Read the model definition and answer for the solid it produces. Units are mm, in the model's axes. A direction names the side the tool comes from. Round coordinates to 2 decimals unless told otherwise and drop trailing zeros. Order: outer loops, then holes, each group sorted by start corner. A loop starts at its lowest first (then second) coordinate and runs counter-clockwise, first axis right, second up. Notation, with made-up numbers: (-11.75, -4.75) - (27.25, -4.75) arc R23 cw to (27.25, 33.25) - close; hole circle Ø8 at (57, 41.5). An arc over 180 degrees is marked (long way). Answer as a JSON object with one key per item and string values. Group by question number.
Q1. A cutting plane is placed at A-A on y = 11.5. Determine the outline of the cut face in (x, z), and give its area (3 significant figures).
Q2. A tool of negligible diameter and unlimited length cuts with its end or side. For faces 1 (the cylindrical face through (18.96, 39.28, 2.99)), 2 (the cylindrical face through (45.36, 37.42, 1.01)), 3 (the flat face through (15.947, 22, 21)), from which of +Z, -Z, +X, -X, +Y, -Y can it reach the whole face along a straight path? Write none if from no direction.
Q3. A cutting plane is placed at D-D on x = 42.5. Determine the outline of the cut face in (y, z), and give its area (3 significant figures).
Q4. A cutting plane is placed at B-B on z = 18.5. Determine the outline of the cut face in (x, y).
Q5. Given pin 1 Ø10 at (x, y) = (43.5, 17.5) entering from +Z; pin 2 Ø3 at (x, y) = (20, 38.5) entering from +Z; pin 3 Ø11 at (x, z) = (40.5, 12.5) entering from -Y, each flat-ended and moving along its own axis, determine where each tip first touches the part or whether it passes through.
Q6. The mould has two halves that part along X. Classify faces 4 (the flat face through (53.947, 23, 20)), 5 (the flat face through (13.947, 23, 20)), 6 (the flat face through (20, 38, 4)): pulls with the +X half, pulls with the -X half, needs draft (parallel to the pull), parting line crosses it, or undercut.
Q7. A cutting plane is placed at C-C on x = 20. Determine the outline of the cut face in (y, z).
Q8. Consider line 1 (X direction, y = 9, z = 5.5); line 2 (Z direction, x = 39, y = 3); line 3 (Y direction, x = 50, z = 11.5). Determine where each line is inside the solid, lowest interval first.
```python
from build123d import *

# Parameters (mm, degrees)
SKETCH_W        = 40
SKETCH_H        = 45
PAD_DEPTH       = 40
SKETCH001_W     = 36
SKETCH001_H     = 46.060933
POCKET_DEPTH    = 38
SKETCH002_R     = 1.4
PAD001_DEPTH    = 2
SKETCH003_R     = 2
POCKET001_DEPTH = 5


with BuildPart() as part:
    # Sketch → Pad (new body)
    with BuildSketch(Plane.XY):
        with Locations((33.946524, 23.135794)):
            Rectangle(SKETCH_W, SKETCH_H)
    extrude(amount=PAD_DEPTH)

    # Sketch001 → Pocket (cut)
    with BuildSketch(Plane.XY.offset(40)):
        with Locations((33.946524, 20.605327)):
            Rectangle(SKETCH001_W, SKETCH001_H)
    extrude(amount=-POCKET_DEPTH, mode=Mode.SUBTRACT)

    # Sketch002 → Pad001 (new body)
    with BuildSketch(Plane.XY.offset(2)):
        with Locations((19.987469, 38.329725)):
            Circle(SKETCH002_R)
        with Locations((47.987469, 6.579725)):
            Circle(SKETCH002_R)
    extrude(amount=PAD001_DEPTH)

    # Sketch003 → Pocket001 (cut)
    with BuildSketch(Plane.XY.offset(2)):
        with Locations((46.946524, 38.635794)):
            Circle(SKETCH003_R)
        with Locations((20.946524, 5.635794)):
            Circle(SKETCH003_R)
    extrude(amount=-POCKET001_DEPTH, mode=Mode.SUBTRACT)


solid = part.part
```
Result set:
{
 "1": {"outline": "(13.95, 0) - (53.95, 0) - (53.95, 40) - (51.95, 40) - (51.95, 2) - (15.95, 2) - (15.95, 40) - (13.95, 40) - close", "area": "232 mm²"},
 "2": {"face 1": "+Z", "face 2": "+Z, -Z", "face 3": "+Z, -Y"},
 "3": {"outline": "(0.64, 0) - (45.64, 0) - (45.64, 40) - (43.64, 40) - (43.64, 2) - (0.64, 2) - close", "area": "166 mm²"},
 "4": {"outline": "(13.95, 0.64) - (15.95, 0.64) - (15.95, 43.64) - (51.95, 43.64) - (51.95, 0.64) - (53.95, 0.64) - (53.95, 45.64) - (13.95, 45.64) - close"},
 "5": {"pin 1": "stops at z = 2", "pin 2": "stops at z = 4", "pin 3": "stops at y = 43.64"},
 "6": {"face 4": "pulls with the +X half", "face 5": "pulls with the -X half", "face 6": "undercut"},
 "7": {"outline": "(0.64, 0) - (3.87, 0) - (3.87, 2) - (0.64, 2) - close; (7.4, 0) - (45.64, 0) - (45.64, 40) - (43.64, 40) - (43.64, 2) - (39.73, 2) - (39.73, 4) - (36.93, 4) - (36.93, 2) - (7.4, 2) - close"},
 "8": {"line 1": "x = 13.95 to 15.95, 51.95 to 53.95", "line 2": "z = 0 to 2", "line 3": "y = 43.64 to 45.64"}
}
